Geometry: final body of the model. Coordinates: model frame, mm. Give positions to 0.01 mm unless a question says otherwise; leave off trailing zeros. Loops run counter-clockwise (first coordinate to the right, second up) from the corner with the lowest first, then second, coordinate; pieces in that order, holes last. Notation, with made-up numbers: M 54,0.25 L 62,0.25 A20 ccw 62,5.25 Z; hole C 12.25,89.5 d5. An arc over 180 degrees is marked long. Put each result on its own line as item: value.
```python
from build123d import *

# Parameters (mm, degrees)
F0_W     = 6.5
F0_H     = 6.5
F1_DEPTH = 1.524
F3_R     = 1.1303
F4_DEPTH = 972


# Not quite as in the source:
# - an extrude ends at something that could not be found from the text; its depth is read off the source's solid


with BuildPart() as f1:
    # F0 (on Front) → F1 (new body)
    with BuildSketch(Plane.XZ):
        Polygon((0, 56.388), (0, 0), (304.8, -5.97408), (304.8, 62.36208), align=None)
        Polygon((304.8, 62.36208), (304.8, -5.97408), (635, -12.446), (635, 68.834), align=None)
        with Locations((467.1477068, -4.4873331716)):
            Rectangle(F0_W, F0_H, mode=Mode.SUBTRACT)
        with Locations((474.1477436, -4.6073838027)):
            Rectangle(F0_W, F0_H, mode=Mode.SUBTRACT)
        with Locations((467.1477068, 4.8497068284)):
            Rectangle(F0_W, F0_H, mode=Mode.SUBTRACT)
        with Locations((474.1477436, 4.7652161973)):
            Rectangle(F0_W, F0_H, mode=Mode.SUBTRACT)
        with Locations((492.8806754, -4.9286535831)):
            Rectangle(F0_W, F0_H, mode=Mode.SUBTRACT)
        with Locations((513.8657236, -5.2885471597)):
            Rectangle(F0_W, F0_H, mode=Mode.SUBTRACT)
        with Locations((533.6728214, -5.628238887)):
            Rectangle(F0_W, F0_H, mode=Mode.SUBTRACT)
        with Locations((492.8806754, 4.5353864169)):
            Rectangle(F0_W, F0_H, mode=Mode.SUBTRACT)
        with Locations((513.8657236, 4.2770928403)):
            Rectangle(F0_W, F0_H, mode=Mode.SUBTRACT)
        with Locations((533.6728214, 4.036461113)):
            Rectangle(F0_W, F0_H, mode=Mode.SUBTRACT)
        with Locations((467.1477068, 14.1867468284)):
            Rectangle(F0_W, F0_H, mode=Mode.SUBTRACT)
        with Locations((474.1477436, 14.1378161973)):
            Rectangle(F0_W, F0_H, mode=Mode.SUBTRACT)
        with Locations((467.1477068, 23.5237868284)):
            Rectangle(F0_W, F0_H, mode=Mode.SUBTRACT)
        with Locations((474.1477436, 23.5104161973)):
            Rectangle(F0_W, F0_H, mode=Mode.SUBTRACT)
        with Locations((492.8806754, 13.9994264169)):
            Rectangle(F0_W, F0_H, mode=Mode.SUBTRACT)
        with Locations((513.8657236, 13.8427328403)):
            Rectangle(F0_W, F0_H, mode=Mode.SUBTRACT)
        with Locations((533.6728214, 13.701161113)):
            Rectangle(F0_W, F0_H, mode=Mode.SUBTRACT)
        with Locations((492.8806754, 23.4634664169)):
            Rectangle(F0_W, F0_H, mode=Mode.SUBTRACT)
        with Locations((513.8657236, 23.4083728403)):
            Rectangle(F0_W, F0_H, mode=Mode.SUBTRACT)
        with Locations((533.6728214, 23.365861113)):
            Rectangle(F0_W, F0_H, mode=Mode.SUBTRACT)
        with Locations((467.1477068, 32.8608268284)):
            Rectangle(F0_W, F0_H, mode=Mode.SUBTRACT)
        with Locations((474.1477436, 32.8830161973)):
            Rectangle(F0_W, F0_H, mode=Mode.SUBTRACT)
        with Locations((467.1477068, 42.1978668284)):
            Rectangle(F0_W, F0_H, mode=Mode.SUBTRACT)
        with Locations((474.1477436, 42.2556161973)):
            Rectangle(F0_W, F0_H, mode=Mode.SUBTRACT)
        with Locations((492.8806754, 32.9275064169)):
            Rectangle(F0_W, F0_H, mode=Mode.SUBTRACT)
        with Locations((513.8657236, 32.9740128403)):
            Rectangle(F0_W, F0_H, mode=Mode.SUBTRACT)
        with Locations((533.6728214, 33.030561113)):
            Rectangle(F0_W, F0_H, mode=Mode.SUBTRACT)
        with Locations((492.8806754, 42.3915464169)):
            Rectangle(F0_W, F0_H, mode=Mode.SUBTRACT)
        with Locations((513.8657236, 42.5396528403)):
            Rectangle(F0_W, F0_H, mode=Mode.SUBTRACT)
        with Locations((533.6728214, 42.695261113)):
            Rectangle(F0_W, F0_H, mode=Mode.SUBTRACT)
        with Locations((467.1477068, 51.5349068284)):
            Rectangle(F0_W, F0_H, mode=Mode.SUBTRACT)
        with Locations((474.1477436, 51.6282161973)):
            Rectangle(F0_W, F0_H, mode=Mode.SUBTRACT)
        with Locations((467.1477068, 60.8719468284)):
            Rectangle(F0_W, F0_H, mode=Mode.SUBTRACT)
        with Locations((474.1477436, 61.0008161973)):
            Rectangle(F0_W, F0_H, mode=Mode.SUBTRACT)
        with Locations((492.8806754, 51.8555864169)):
            Rectangle(F0_W, F0_H, mode=Mode.SUBTRACT)
        with Locations((513.8657236, 52.1052928403)):
            Rectangle(F0_W, F0_H, mode=Mode.SUBTRACT)
        with Locations((533.6728214, 52.359961113)):
            Rectangle(F0_W, F0_H, mode=Mode.SUBTRACT)
        with Locations((492.8806754, 61.3196264169)):
            Rectangle(F0_W, F0_H, mode=Mode.SUBTRACT)
        with Locations((513.8657236, 61.6709328403)):
            Rectangle(F0_W, F0_H, mode=Mode.SUBTRACT)
        with Locations((533.6728214, 62.024661113)):
            Rectangle(F0_W, F0_H, mode=Mode.SUBTRACT)
    extrude(amount=F1_DEPTH)

    # F3 (on face) → F4 (cut, through all)
    with BuildSketch(Plane.XZ.offset(1.524)):
        with Locations((97.3946236, 8.0847413075)):
            Circle(F3_R)
        with Locations((3.175, 8.1216754)):
            Circle(F3_R)
        with Locations((181.3279076, 8.0518394602)):
            Circle(F3_R)
        with Locations((290.391088, 8.0090866935)):
            Circle(F3_R)
        with Locations((409.2984448, 7.9624750096)):
            Circle(F3_R)
        with Locations((524.05534, 7.9174903067)):
            Circle(F3_R)
        with Locations((624.435886, 7.8781411327)):
            Circle(F3_R)
        with Locations((97.3946236, 48.3032586925)):
            Circle(F3_R)
        with Locations((3.175, 48.2663246)):
            Circle(F3_R)
        with Locations((181.3279076, 48.3361605398)):
            Circle(F3_R)
        with Locations((290.391088, 48.3789133065)):
            Circle(F3_R)
        with Locations((409.2984448, 48.4255249904)):
            Circle(F3_R)
        with Locations((524.05534, 48.4705096933)):
            Circle(F3_R)
        with Locations((624.435886, 48.5098588673)):
            Circle(F3_R)
    extrude(amount=F4_DEPTH, mode=Mode.SUBTRACT)


solid = f1.part
```
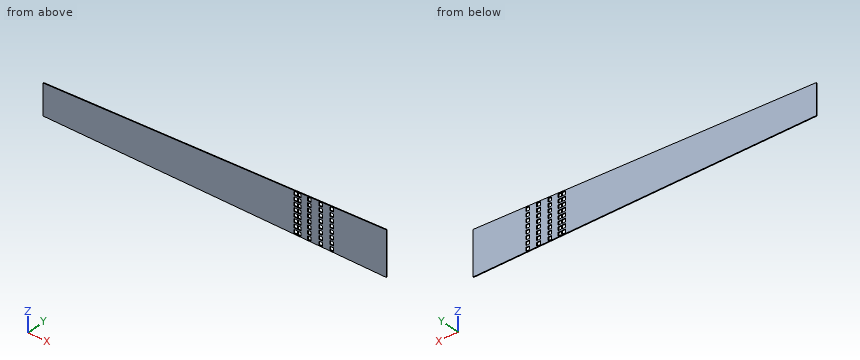
Item 1: Section A-A on y = -0.65. Count the separate pieces of the cut face and the enclosed holes in it, then the cut area to 3 significant figures.
Output values:
separate pieces: 1
enclosed holes: 40
area: 42,000 mm²
Item 2: Pin query (flat end, axial travel): pin 1 Ø0.5 at (x, y) = (492.5, -1) entering from +Z; pin 2 Ø0.8 at (x, y) = (532.5, -1) entering from -Z; pin 3 Ø0.8 at (x, y) = (514.5, -0.5) entering from +Z. Return the tip coordinate at first contact, or that it passes through.
Output values:
pin 1: z = 66.05
pin 2: z = -10.44
pin 3: z = 66.48
Item 3: Line query: probe 1 along X at (y, z) = (-0.05, 13.5); probe 2 along Z at (x, y) = (422, -1.3); probe 3 along Z at (x, y) = (449.5, -1.3). Output: solid intervals per line, ascending. Write a range as [from, to].
Output values:
probe 1: [0, 463.9], [470.4, 470.9], [477.4, 489.63], [496.13, 510.62], [517.12, 530.42], [536.92, 635]
probe 2: [-8.27, 64.66]
probe 3: [-8.81, 65.2]
Item 4: Section C-C on x = 125.5. Output: boundary loops of the cut face in (y, z), then the cut area to 3 significant figures.
Output values:
outline: M -1.52,-2.46 L 0,-2.46 L 0,58.85 L -1.52,58.85 Z
area: 93.4 mm²
Item 5: Section B-B on x = 438.5. Output: boundary loops of the cut face in (y, z), then the cut area to 3 significant figures.
Output values:
outline: M -1.52,-8.59 L 0,-8.59 L 0,64.98 L -1.52,64.98 Z
area: 112 mm²
